Geometry check sheet. Reference: the model listing, model coordinates, mm. Face numbers are marked on the shaded views. A direction names the side the tool comes from. Give positions to 0.01 mm unless a question says otherwise; leave off trailing zeros. Loops run counter-clockwise (first coordinate to the right, second up) from the corner with the lowest first, then second, coordinate; pieces in that order, holes last.
1. Cross-section at A-A, the plane z = 19. Record the cut outline in (x, y).
2. Cross-section at C-C, the plane z = 36.5. Record the cut outline in (x, y), plus the area to 3 significant figures.
3. Cross-section at B-B, the plane x = 10. Record the cut outline in (y, z).
4. Material ranges on L1, parallel to Y at x = 8.75, z = 18; L2, parallel to Z at x = 17.75, y = 32.5; L3, parallel to Y at x = 11.5, z = 37, recorded low to high.
5. Release check for a two-part mould opening along Z. For the marked faces 5, 6 and 7 record: +Z half, -Z half, draft (parallel to the pull), parting line (faces both ways), or undercut.
6. Go/stop test with flat-tipped pins: pin 1 Ø1.5 at (x, z) = (17, 36) entering from -Y; pin 2 Ø11 at (x, z) = (11, 17.5) entering from +Y. Record where each tip stops, or that it passes through.
7. Tool access check on the marked faces 1, 2, 3 and 4. Record the directions out of +Z, -Z, +X, -X, +Y, -Y that give a thin tool (end or side, any length) a straight path to the whole face; none if there is none.
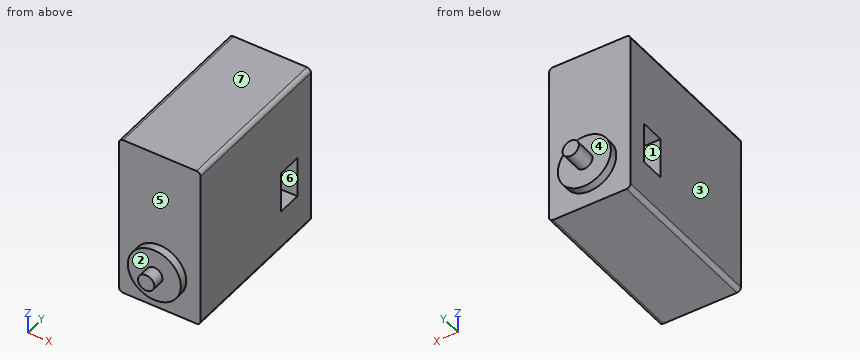
Autodesk Inventor part; units mm, degrees
ref_plane "YZ Plane" through (0, 0, 0) normal (1, 0, 0) x (0, 1, 0)
ref_plane "XZ Plane" through (0, 0, 0) normal (0, 1, 0) x (-1, 0, 0)
ref_plane "XY Plane" through (0, 0, 0) normal (0, 0, 1) x (1, 0, 0)
sketch "Sketch1" plane through (0, 0, 0) normal (0, 0, 1) x (1, 0, 0)
  line L0 (0, 0) -> (0, 40.5)
  line L1 (0, 40.5) -> (20, 40.5)
  line L2 (20, 40.5) -> (20, 0)
  line L3 (20, 0) -> (0, 0)
  dimension "d0" = 40.5
  dimension "d1" = 20
extrude "Extrusion1" add sketch "Sketch1" along normal blind 40
sketch "Sketch2" plane through (0, 40.5, 0) normal (0, 1, 0) x (1, 0, 0)
  line L0 (20, 0) -> (0, 0)
  line L1 (10, 0) -> (10, -10)
  circle A0 centre (10, -10) radius 5
  dimension "d4" = 10
  dimension "d5" = 10
extrude "Extrusion2" add sketch "Sketch2" along normal blind 1
sketch "Sketch3" plane through (10, 41.5, 10) normal (0, 1, 0) x (1, 0, 0)
  circle A0 centre (0, 0) radius 2
  point P0 (-10, 10)
  dimension "d8" = 4
extrude "Extrusion3" add sketch "Sketch3" along normal blind 6
fillet "Fillet1" radius 1 4 edges at (0, 20.25, 40) (20, 20.25, 40) (20, 20.25, 0) (0, 20.25, 0)
sketch "Sketch4" plane through (1, 0, 0) normal (0, -1, 0) x (1, 0, 0)
  line L0 (18, 0) -> (0, 0)
  line L1 (9, 0) -> (9, 10)
  circle A0 centre (9, 10) radius 5
  point P0 (-1, 0)
  dimension "d12" = 10
  dimension "d13" = 10
extrude "Extrusion4" add sketch "Sketch4" along normal blind 1
sketch "Sketch5" plane through (10, -1, 10) normal (0, -1, 0) x (1, 0, 0)
  circle A0 centre (0, 0) radius 2
  point P0 (-10, -10)
  dimension "d16" = 4
extrude "Extrusion5" add sketch "Sketch5" along normal blind 4
sketch "Boceto6" plane through (0, 0, 1) normal (-1, 0, 0) x (0, 0, 1)
  line L0 (-1, 0) -> (-1, 40.5)
  line L1 (-1, 40.5) -> (-1, 35.5)
  line L2 (-1, 35.5) -> (9, 35.5)
  line L3 (9, 35.5) -> (9, 29.5)
  line L4 (9, 29.5) -> (19, 29.5)
  line L5 (19, 29.5) -> (19, 35.5)
  line L6 (19, 35.5) -> (9, 35.5)
  dimension "d19" = 5
  dimension "d20" = 10
  dimension "d21" = 6
  dimension "d22" = 10
extrude "Extrusión6" cut sketch "Boceto6" against normal up to next
sketch "Boceto7" plane through (1, 0, 0) normal (0, -1, 0) x (1, 0, 0)
  line L0 (-1, 10) -> (19, 10)
  circle A0 centre (9, 10) radius 6.5
  circle A1 centre (9, 10) radius 2
  point P0 (-1, 0)
  dimension "d25" = 13
extrude "Extrusión8" add sketch "Boceto7" along normal blind 2 contours A1 L0 A0 | L0 A0 A1
sketch "Boceto8" plane through (1, 40.5, 0) normal (0, 1, 0) x (1, 0, 0)
  circle A0 centre (9, -10) radius 2
  circle A1 centre (9, -10) radius 6.5
  circle A2 centre (9, -10) radius 6.5
  circle A3 centre (9, -10) radius 2
  point P0 (-1, 0)
  dimension "d30" = 13
extrude "Extrusión9" add sketch "Boceto8" along normal blind 2
properties part number "servo_FT_SC"
Result:
1. outline: (0, 0) - (20, 0) - (20, 29.5) - (0, 29.5) - close; (0, 35.5) - (20, 35.5) - (20, 40.5) - (0, 40.5) - close
2. outline: (0, 0) - (20, 0) - (20, 40.5) - (0, 40.5) - close
2. area: 810 mm2
3. outline: (-5, 8) - (-2, 8) - (-2, 3.5) - (0, 3.5) - (0, 0) - (40.5, 0) - (40.5, 3.5) - (42.5, 3.5) - (42.5, 8) - (47.5, 8) - (47.5, 12) - (42.5, 12) - (42.5, 16.5) - (40.5, 16.5) - (40.5, 40) - (0, 40) - (0, 16.5) - (-2, 16.5) - (-2, 12) - (-5, 12) - close; hole (29.5, 10) - (35.5, 10) - (35.5, 20) - (29.5, 20) - close
4. L1: y = 0 to 29.5, 35.5 to 40.5
4. L2: z = 0 to 10, 20 to 40
4. L3: y = 0 to 40.5
5. face 5: draft
5. face 6: undercut
5. face 7: +Z half
6. pin 1: stops at y = 0
6. pin 2: stops at y = 42.5
7. face 1: +X, -X
7. face 2: -Y
7. face 3: +Z, -Z, -X, +Y, -Y
7. face 4: +Y
